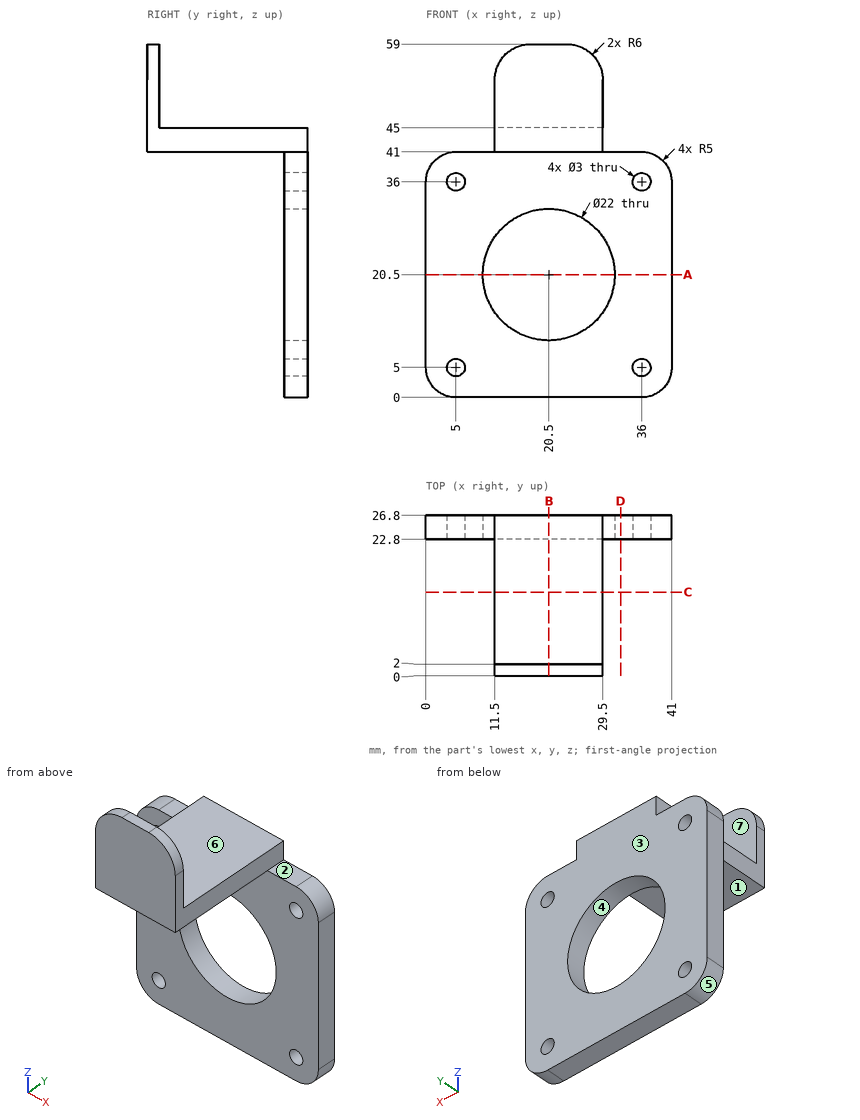
Source: three-view drawing plus pictorial views. Frame: mm from the lowest corner of the part. A direction names the side the tool comes from. Round coordinates to 2 decimals unless told otherwise and drop trailing zeros. Order: outer loops, then holes, each group sorted by start corner. A loop starts at its lowest first (then second) coordinate and runs counter-clockwise, first axis right, second up. Notation, with made-up numbers: (20.5, -31) -> (39.5, -31) arc R11 ccw to (39.5, -23) -> close; hole circle Ø4 at (-5, 32.25). An arc over 180 degrees is marked (long way). Use one line per item in the form item = value.
(1) Section D-D on x = 32.5. Return loops of the section in (y, z).
Results list:
outline = (22.8, 0) -> (26.8, 0) -> (26.8, 41) -> (22.8, 41) -> close
(2) Section A-A on z = 20.5. Return loops of the section in (x, y).
Results list:
outline = (0, 22.8) -> (9.5, 22.8) -> (9.5, 26.8) -> (0, 26.8) -> close; (31.5, 22.8) -> (41, 22.8) -> (41, 26.8) -> (31.5, 26.8) -> close
(3) Access query for the marked faces 1, 2 and 3. Directions: +Z, -Z, +X, -X, +Y, -Y. A direction counts if a zero-diameter tool reaches every point of the face in a straight line with its end or side. Return the directions, or none.
Results list:
face_1 = -Z, +X, -X, -Y
face_2 = +Z, +X, +Y, -Y
face_3 = +Z, -Z, +X, -X, +Y
(4) Section B-B on x = 20.5. Return loops of the section in (y, z), and give its area (3 significant figures).
Results list:
outline = (0, 41) -> (22.8, 41) -> (22.8, 31.5) -> (26.8, 31.5) -> (26.8, 45) -> (2, 45) -> (2, 59) -> (0, 59) -> close; (22.8, 0) -> (26.8, 0) -> (26.8, 9.5) -> (22.8, 9.5) -> close
area = 211 mm^2
(5) First-contact query: pin 1 Ø2.5 at (x, z) = (5, 36) entering from +Y; pin 2 Ø5 at (x, z) = (36, 36) entering from -Y; pin 3 Ø12 at (x, y) = (24.5, 19) entering from +Z; pin 4 Ø1.2 at (x, y) = (9.5, 25.5) entering from +Z. Flat tips, straight axial feed; report the tip coordinate or a pass-through.
Results list:
pin_1 = through
pin_2 = 22.8
pin_3 = 45
pin_4 = 41
(6) Ray query, probe 1 along X at (y, z) = (24.8, 5); probe 2 along Y at (x, z) = (15, 55); probe 3 along Y at (x, z) = (37.5, 21). Return the intervals inside material, ascending. Write a range as [from, to].
Results list:
probe_1 = [0, 3.5], [6.5, 34.5], [37.5, 41]
probe_2 = [0, 2]
probe_3 = [22.8, 26.8]
(7) Draft query along Z for the marked faces 4, 5, 6 and 7. Return one class per face: pulls with the +Z half, pulls with the -Z half, needs draft (parallel to the pull), parting line crosses it, or undercut.
Results list:
face_4 = undercut
face_5 = pulls with the -Z half
face_6 = pulls with the +Z half
face_7 = needs draft
(8) Section C-C on y = 14. Return loops of the section in (x, z), and give its area (3 significant figures).
Results list:
outline = (11.5, 41) -> (29.5, 41) -> (29.5, 45) -> (11.5, 45) -> close
area = 72.0 mm^2
